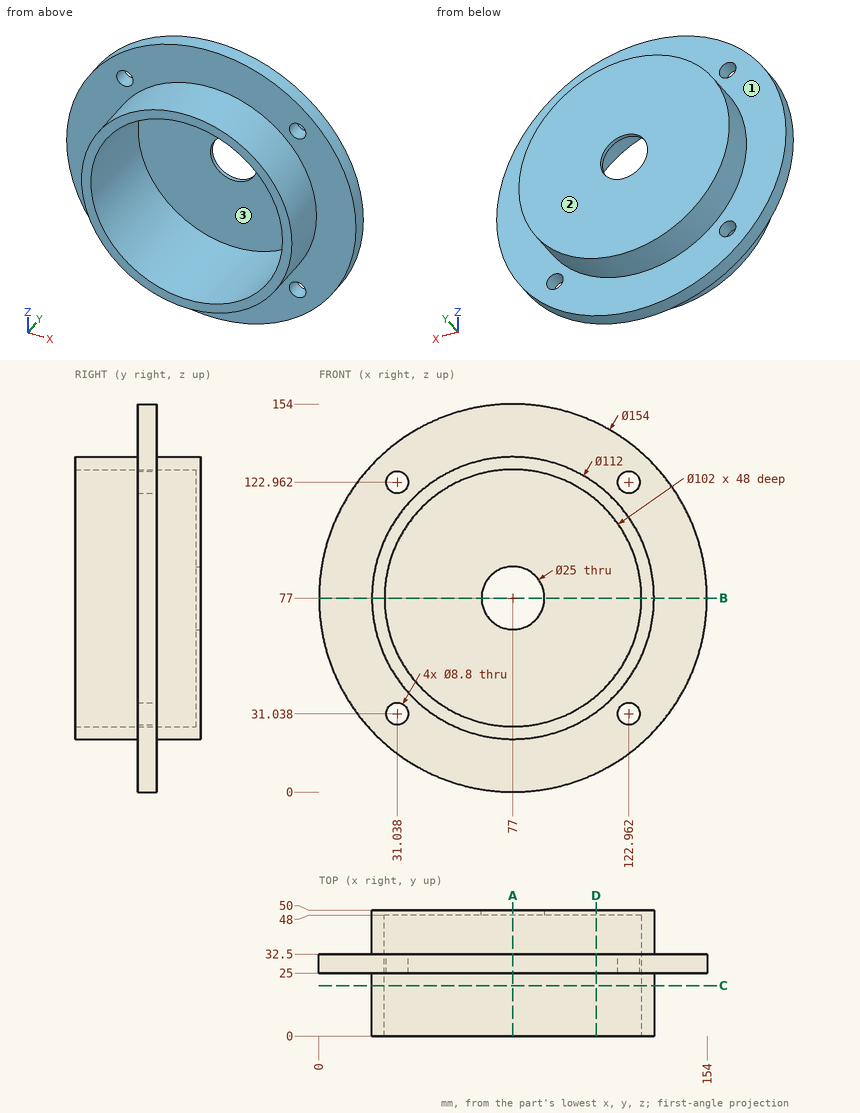
Design review of the part shown in the three views and the two pictorial views. Dimensions are in mm from the part's minimum x, y and z. A direction names the side the tool comes from. Round coordinates to 2 decimals unless told otherwise and drop trailing zeros. Write each loop counter-clockwise with the first axis right and the second up, starting at its lowest first coordinate (ties: lowest second). Pieces come first, ordered by that corner, then holes.
Item 1: Clearance check with flat-ended pins moving along their axes: pin 1 Ø4 at (x, y) = (31.5, 22.5) entering from +Z; pin 2 Ø10 at (x, z) = (122.96, 122.96) entering from -Y; pin 3 Ø5 at (x, y) = (109.5, 21) entering from -Z. State where each tip first meets the part, or that it passes through.
Item 2: We need section D-D on x = 110. Write out the cut boundary in (y, z), and give its area (3 significant figures).
Item 3: We need section A-A on x = 77. Write out the cut boundary in (y, z), and give its area (3 significant figures).
Item 4: For the marked faces 1, 2 and 3, list the 3-axis set-ups (+Z, -Z, +X, -X, +Y, -Y) from which the entire face can be reached by the end or side of a thin tool; tool diameter is ignored.
Item 5: We need section C-C on y = 20. Write out the cut boundary in (x, z).
Item 6: For probe 1 along Z at (x, y) = (77, 36.5); probe 2 along Y at (x, z) = (65, 143); probe 3 along Y at (x, z) = (94, 56), list the stretches that pass through material, from the lowest coordinate up.
Item 7: We need section B-B on z = 77. Write out the cut boundary in (x, y).
Returned:
1. pin 1: stops at z = 112.27
1. pin 2: stops at y = 25
1. pin 3: stops at z = 29.71
2. outline: (0, 31.76) - (25, 31.76) - (25, 7.43) - (32.5, 7.43) - (32.5, 31.76) - (50, 31.76) - (50, 122.24) - (32.5, 122.24) - (32.5, 146.57) - (25, 146.57) - (25, 122.24) - (0, 122.24) - (0, 115.88) - (48, 115.88) - (48, 38.12) - (0, 38.12) - close
2. area: 1,160 mm2
3. outline: (0, 21) - (25, 21) - (25, 0) - (32.5, 0) - (32.5, 21) - (50, 21) - (50, 64.5) - (48, 64.5) - (48, 26) - (0, 26) - close; (0, 128) - (48, 128) - (48, 89.5) - (50, 89.5) - (50, 133) - (32.5, 133) - (32.5, 154) - (25, 154) - (25, 133) - (0, 133) - close
3. area: 969 mm2
4. face 1: +Y
4. face 2: +Z, -Z, +X, -X, +Y
4. face 3: -Y
5. outline: circle Ø112 at (77, 77); hole circle Ø102 at (77, 77)
6. probe 1: z = 21 to 26, 128 to 133
6. probe 2: y = 25 to 32.5
6. probe 3: y = 48 to 50
7. outline: (0, 25) - (21, 25) - (21, 0) - (26, 0) - (26, 48) - (64.5, 48) - (64.5, 50) - (21, 50) - (21, 32.5) - (0, 32.5) - close; (89.5, 48) - (128, 48) - (128, 0) - (133, 0) - (133, 25) - (154, 25) - (154, 32.5) - (133, 32.5) - (133, 50) - (89.5, 50) - close
